from build123d import *

# Parameters (mm, degrees)
BOX_W     = 100
BOX_H     = 40
BOX_DEPTH = 100


with BuildPart() as cube:
    # Box → Box (new body)
    with BuildSketch(Plane(origin=(4896, -20, -56), x_dir=(1, 0, 0), z_dir=(0, 0, 1))):
        with Locations((50, 20)):
            Rectangle(BOX_W, BOX_H)
    extrude(amount=BOX_DEPTH)


with BuildPart() as cut:
    # Sweep: sweep along a path in Sketch001
    with BuildLine(Plane.YZ) as sweep_path:
        Line((50, -102.428871), (-50, -102.428871))
    # Sketch → Sweep (sweep)
    with BuildSketch(Plane.XZ):
        with BuildLine():
            Line((5079.153809, -307.963104), (4972.606463, 10.450841))
            ThreePointArc((4972.606463, 10.450841), (4938.873384, 33.689038), (4907.556965, 7.284185))
            Line((4907.556965, 7.284185), (4907.556965, -308.010559))
            add(Edge.make_bspline(
                [(4907.556965, -308.010559), (4907.383301, -349.562683), (5004.027832, -362.999908), (5078.214844, -516.165161)],
                knots=[0, 0, 0, 0, 1, 1, 1, 1], degree=3))
            Line((5078.214844, -516.165161), (5079.153809, -307.963104))
        make_face()
    sweep(path=sweep_path.line)

    # Cut: cut Cube
    add(cube.part, mode=Mode.SUBTRACT)


solid = cut.part
The model under review builds one solid part; all positions refer to its coordinate system, in mm. A direction names the side the tool comes from. Coordinates: 2 decimals unless noted, no trailing zeros. Order: outer loops, then holes, each group sorted by start corner. A loop starts at its lowest first (then second) coordinate and runs counter-clockwise, first axis right, second up. Notation, with made-up numbers: (0.5, 70.25) -> (31.5, 70.25) arc R33 cw to (31.5, 108.25) -> close; hole circle Ø8 at (20.25, 25.25). An arc over 180 degrees is marked (long way). Answer in a Markdown table with one row per item.
(1) Machinability: for faces 4 (the flat face through (4907.557, -1, -148)), 5 (the flat face through (4941, -20, -22)), which of the approach directions +Z, -Z, +X, -X, +Y, -Y give a long, thin tool a straight path to every point of the face, cutting with its end or side? Answer none if there is none.
Answers:
| item | result |
|---|---|
| face 4 | +Z, -Z, -X, +Y, -Y |
| face 5 | +Z, +X, -X |
(2) Consider section C-C (z = -134). Write out the cut boundary in (x, y), plus the area to 3 significant figures.
Answers:
| item | result |
|---|---|
| outline | (4907.56, -50) -> (5020.94, -50) -> (5020.94, 50) -> (4907.56, 50) -> close |
| area | 11,300 mm² |
(3) Insertion check: pin 1 (10 mm diameter, centred on x = 5039.5, y = 33.5, fed in from -Z); pin 2 (2 mm diameter, centred on y = 21, z = -160.5, fed in from +X); pin 3 (2 mm diameter, centred on y = -18, z = -443.5, fed in from -X). Each pin has a flat end and moves straight along its axis. Give the tip position at first contact, or say it passes through.
Answers:
| item | result |
|---|---|
| pin 1 | z = -457.26 |
| pin 2 | x = 5030.14 |
| pin 3 | x = 5034.06 |
(4) The part is to be moulded in two halves that separate along Y. For faces 1 (the flat face through (4951, 0, -56)), 2 (the flat face through (4994, 50, -237)), 3 (the flat face through (4994, -50, -237)), say which applies: +Y half, -Y half, draft (parallel to the pull), parting line (faces both ways), or undercut.
Answers:
| item | result |
|---|---|
| face 1 | undercut |
| face 2 | +Y half |
| face 3 | -Y half |
(5) Consider section B-B (z = -232). Write out the cut boundary in (x, y), plus the area to 3 significant figures.
Answers:
| item | result |
|---|---|
| outline | (4907.56, -50) -> (5053.74, -50) -> (5053.74, 50) -> (4907.56, 50) -> close |
| area | 14,600 mm² |
(6) Wall thickness on line 1 along Y through (x, z) = (4939.5, -43); line 2 along X through (y, z) = (-30, -368); line 3 along Z through (x, y) = (4964, -17): over which ranges is each line inside the solid? List them lowest first.
Answers:
| item | result |
|---|---|
| line 1 | -50 to -20, 20 to 50 |
| line 2 | 4962.29 to 5078.88 |
| line 3 | -369.41 to -56 |
(7) Consider section A-A (z = -43.5). Write out the cut boundary in (x, y), plus the area to 3 significant figures.
Answers:
| item | result |
|---|---|
| outline | (4907.56, -50) -> (4990.66, -50) -> (4990.66, -20) -> (4907.56, -20) -> close; (4907.56, 20) -> (4990.66, 20) -> (4990.66, 50) -> (4907.56, 50) -> close |
| area | 4,990 mm² |
